Drawing for the job (mm, zero at the part's lowest x, y, z). Round coordinates to 2 decimals unless told otherwise and drop trailing zeros. Loops run counter-clockwise (first coordinate to the right, second up) from the corner with the lowest first, then second, coordinate; pieces in that order, holes last. Notation, with made-up numbers: M 81.5,76.5 L 104.5,76.5 A21 cw 104.5,86.5 Z; hole C 13.5,17.25 d7. An arc over 180 degrees is marked long. Use a Markdown table: item, result. Add a question column.
Q1. Pin check, flat tips, straight feed: pin 1 (2.5 mm diameter, centred on y = 4, z = 1.5, fed in from -X); pin 2 (1.5 mm diameter, centred on x = 81, y = 7.5, fed in from +Z); pin 3 (1.5 mm diameter, centred on y = 4, z = 2.5, fed in from +X). Stop position of each tip, or through.
Q2. Cut at A-A (x = 50.5). Give the cut face in (y, z).
Q3. Cut at B-B (z = 2.5). Give the cut face in (x, y).
Q4. Probe line 1 (X direction, y = 12.5, z = 4.55); line 2 (X direction, y = 12.25, z = 1.5); line 3 (Y direction, x = 154, z = 3.5). List the from-to ranges inside material, lowest first. Write a range as from..to.
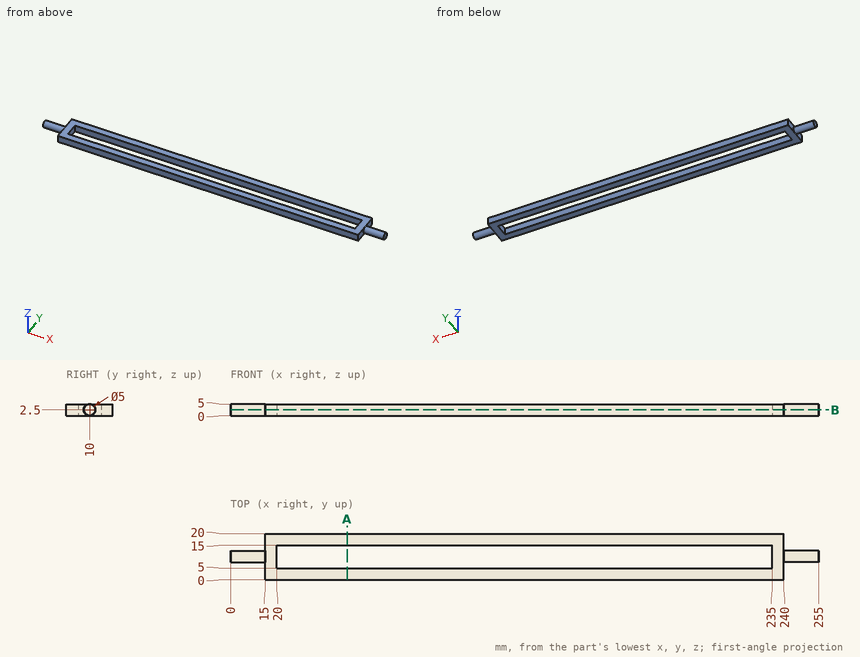
Checked values:
| question | item | result |
|---|---|---|
| 1 | pin 1 | stops at x = 15 |
| 1 | pin 2 | passes through |
| 1 | pin 3 | stops at x = 240 |
| 2 | outline | M 0,0 L 5,0 L 5,5 L 0,5 Z; M 15,0 L 20,0 L 20,5 L 15,5 Z |
| 3 | outline | M 0,7.5 L 15,7.5 L 15,0 L 240,0 L 240,7.5 L 255,7.5 L 255,12.5 L 240,12.5 L 240,20 L 15,20 L 15,12.5 L 0,12.5 Z; hole M 20,5 L 235,5 L 235,15 L 20,15 Z |
| 4 | line 1 | x = 15..20, 235..240 |
| 4 | line 2 | x = 0..20, 235..255 |
| 4 | line 3 | y = 0..5, 15..20 |
